```python
from build123d import *

# Parameters (mm, degrees)
MODEL_R             = 25
BOSS_EXTRUDE1_DEPTH = 6
BOSS_EXTRUDE2_START = -6
SKETCH2_R           = 45
SKETCH2_R_2         = 25
BOSS_EXTRUDE2_DEPTH = 6


with BuildPart() as part:
    # Model → Boss-Extrude1 (new body)
    with BuildSketch(Plane.XY):
        with Locations((642.3, -192)):
            Circle(MODEL_R)
        Polygon((628.8, -184.205771366), (628.8, -199.794228634), (642.3, -207.588457268), (655.8, -199.794228634), (655.8, -184.205771366), (642.3, -176.411542732), align=None, mode=Mode.SUBTRACT)
    extrude(amount=BOSS_EXTRUDE1_DEPTH)

    # Sketch2 → Boss-Extrude2 (add)
    with BuildSketch(Plane.XY.offset(6).offset(BOSS_EXTRUDE2_START)):
        with Locations((642.3, -192)):
            Circle(SKETCH2_R)
        with Locations((642.3, -192)):
            Circle(SKETCH2_R_2, mode=Mode.SUBTRACT)
    extrude(amount=BOSS_EXTRUDE2_DEPTH)


solid = part.part
```
Part model, mm, in its own coordinate system. A direction names the side the tool comes from. Round coordinates to 2 decimals unless told otherwise and drop trailing zeros. Write each loop counter-clockwise with the first axis right and the second up, starting at its lowest first coordinate (ties: lowest second). Pieces come first, ordered by that corner, then holes. Notation, with made-up numbers: M 60,-31 L 107,-31 A22 cw 107,-12 Z; hole C -24.5,1 d7. An arc over 180 degrees is marked long. Answer as CSV lines item,"result". Start each with the question number.
1) Drop flat-ended pins along their axis: pin 1 (2 mm diameter, centred on x = 607, z = 3, fed in from -Y); pin 2 (3 mm diameter, centred on y = -189.5, z = 1.5, fed in from -X); pin 3 (1 mm diameter, centred on y = -219, z = 4, fed in from -X). Give the stop position or say it passes through.
2) Band-saw the part on D-D (x = 667.5). List the corners of the cut face in (y, z).
3) Band-saw the part on A-A (y = -192). List the corners of the cut face in (x, z), then the cut area to 3 significant figures.
4) Drill centre lines: L1, parallel to X at y = -205.5, z = 0.55; L2, parallel to X at y = -195.5, z = 0.85; L3, parallel to Y at x = 640, z = 2.85. Where is each one in solid material? Low to high.
5) Band-saw the part on C-C (x = 631.5). List the corners of the cut face in (y, z), then the cut area to 3 significant figures.
6) Which spindle directions (+Z, -Z, +X, -X, +Y, -Y) get a long thin tool onto all of the face, cutting with end or side? Do faces 1 (the face through (652, -181, 0)), 2 (the face through (649.14, -180.36, 2.96)). Say none if no direction does.
7) Band-saw the part on B-B (z = 3.2). List the corners of the cut face in (x, y), then the cut area to 3 significant figures.
8) Mould opens along X. For faces 3 (the face through (635.46, -203.64, 2.96)), 4 (the face through (652, -181, 6)), 5 (the face through (597.344, -190.021, 2.958)) say: +X half, -X half, draft (parallel to the pull), parting line (faces both ways), or undercut.
Worked out:
1,pin 1,"y = -221.13"
1,pin 2,"x = 597.31"
1,pin 3,"x = 605.93"
2,outline,"M -229.28,0 L -154.72,0 L -154.72,6 L -229.28,6 Z"
3,outline,"M 597.3,0 L 628.8,0 L 628.8,6 L 597.3,6 Z; M 655.8,0 L 687.3,0 L 687.3,6 L 655.8,6 Z"
3,area,"378 mm²"
4,L1,"599.37 to 638.68, 645.92 to 685.23"
4,L2,"597.44 to 628.8, 655.8 to 687.16"
4,L3,"-236.94 to -206.26, -177.74 to -147.06"
5,outline,"M -235.68,0 L -201.35,0 L -201.35,6 L -235.68,6 Z; M -182.65,0 L -148.32,0 L -148.32,6 L -182.65,6 Z"
5,area,"412 mm²"
6,face 1,"-Z, +X, -X, +Y, -Y"
6,face 2,"+Z, -Z"
7,outline,"C 642.3,-192 d90; hole M 628.8,-199.79 L 642.3,-207.59 L 655.8,-199.79 L 655.8,-184.21 L 642.3,-176.41 L 628.8,-184.21 Z"
7,area,"5,730 mm²"
8,face 3,"undercut"
8,face 4,"draft"
8,face 5,"parting line"
